```python
from build123d import *

# Parameters (mm, degrees)
F0_R     = 1.5
F1_DEPTH = 5
F2_DEPTH = 268
F3_R     = 1.65
F3_R_2   = 1.35
F4_DEPTH = 5.001
F5_W     = 12
F5_H     = 2
F6_DEPTH = 12
F7_DEPTH = 5
F8_R     = 1.65
F9_DEPTH = 52.0010001044


# Not quite as in the source:
# - an extrude ends at something that could not be found from the text; its depth is read off the source's solid


with BuildPart() as f1:
    # F0 (on Top) → F1 (new body)
    with BuildSketch(Plane.XY):
        Polygon((-52.0408339798, -45.9276453106), (-151.9144345724, -45.9276453106), (-151.9144345724, -55.9276454151), (-45.8887560524, -55.9276454151), (-25.683571109, -15.9276453106), (9.5701563833, -15.9276453106), (11.0855654276, -12.9276453106), (44.264588505, -12.9276453106), (44.264588505, -5.9276453106), (27.9570557177, -5.9276453106), (-31.8356490892, -5.9276453106), (-31.9144345724, -6.0836161342), align=None)
        with Locations((-136.9144345724, -50.9276454151)):
            Circle(F0_R, mode=Mode.SUBTRACT)
        with Locations((-96.9144345724, -50.9276454151)):
            Circle(F0_R, mode=Mode.SUBTRACT)
        with Locations((-76.9144345724, -50.9276454151)):
            Circle(F0_R, mode=Mode.SUBTRACT)
    extrude(amount=F1_DEPTH)

    # F0 (on Top) → F2 (cut, through all)
    with BuildSketch(Plane.XY):
        with Locations((-76.9144345724, -50.9276454151)):
            Circle(F0_R)
        with Locations((-96.9144345724, -50.9276454151)):
            Circle(F0_R)
    extrude(amount=-F2_DEPTH, mode=Mode.SUBTRACT)

    # F3 (on face) → F4 (cut, through all)
    with BuildSketch(Plane.XY.offset(5)):
        with Locations((39.264588505, -9.4276453106)):
            Circle(F3_R)
        with Locations((19.264588505, -9.4276453106)):
            Circle(F3_R_2)
        with Locations((-33.3638369572, -20.042586615)):
            Circle(F3_R)
        with Locations((-46.4391469312, -45.9276454151)):
            Circle(F3_R)
    extrude(amount=-F4_DEPTH, mode=Mode.SUBTRACT)

    # F5 (on face) → F6 (join)
    with BuildSketch(Plane.XY.offset(5)):
        with Locations((-58.9144345724, -54.9276454151)):
            Rectangle(F5_W, F5_H)
        with Locations((-58.9144345724, -56.9276454151)):
            Rectangle(F5_W, F5_H)
    extrude(amount=F6_DEPTH)

    # F7 (add): a face of the model
    f7_faces = [f1.faces().sort_by_distance(p)[0] for p in [
        (-58.9144345724, -56.9276454151, 5),
    ]]
    extrude(f7_faces, amount=F7_DEPTH)

    # F8 (on face) → F9 (cut, through all)
    with BuildSketch(Plane.XZ.offset(57.9276454151)):
        with Locations((-58.9144345724, 11)):
            Circle(F8_R)
    extrude(amount=-F9_DEPTH, mode=Mode.SUBTRACT)


solid = f1.part
```
Model file for the job. Use its own axes, mm. A direction names the side the tool comes from. Give positions to 0.01 mm unless a question says otherwise; leave off trailing zeros. Order: outer loops, then holes, each group sorted by start corner. A loop starts at its lowest first (then second) coordinate and runs counter-clockwise, first axis right, second up.
1) Pin check, flat tips, straight feed: pin 1 (1.5 mm diameter, centred on x = 27.5, z = 2, fed in from -Y); pin 2 (4 mm diameter, centred on y = -43.5, z = 7.5, fed in from -X); pin 3 (1.5 mm diameter, centred on x = -14.5, z = 3.5, fed in from -Y); pin 4 (2 mm diameter, centred on y = -57, z = 11.5, fed in from +X). Stop position of each tip, or through.
2) Mould opens along Y. For faces 1 (the flat face through (-49, -55.928, 2)), 2 (the flat face through (7, -5.928, 2)), 3 (the cylindrical face through (-48.088, -45.855, 2.535)) say: +Y half, -Y half, draft (parallel to the pull), parting line (faces both ways), or undercut.
3) Saw through at A-A, the plane z = 11. Write the cut outline in (x, y), then the cut area to 3 significant figures.
4) Saw through at C-C, the plane x = -18.5. Write the cut outline in (y, z), then the cut area to 3 significant figures.
5) Saw through at D-D, the plane y = -27. Write the cut outline in (x, z).
6) 3-axis set-ups, long thin cutter, end or side, ignore diameter. For faces 4 (the flat face through (-59, -56, 17)), 5 (the flat face through (27, -12.928, 2)), 6 (the flat face through (-109, -55.928, 2)), 7 (the cylindrical face through (-34.67, -21.05, 2.54)), 8 (the flat face through (-101, -45.928, 2)): which of +Z, -Z, +X, -X, +Y, -Y reach the whole face in a straight line?
7) Wall check: probe 1 along Z at (x, y) = (-102, -46); probe 2 along X at (y, z) = (-54, 15.5); probe 3 along Y at (x, z) = (-55, 10.25). Give the ranges that are in metal, low to high.
8) Saw through at B-B, the plane z = 2.75. Write the cut outline in (x, y).
Computed:
1. pin 1: stops at y = -12.93
1. pin 2: passes through
1. pin 3: stops at y = -15.93
1. pin 4: stops at x = -52.91
2. face 1: -Y half
2. face 2: +Y half
2. face 3: undercut
3. outline: (-64.91, -57.93) - (-60.56, -57.93) - (-60.56, -53.93) - (-64.91, -53.93) - close; (-57.26, -57.93) - (-52.91, -57.93) - (-52.91, -53.93) - (-57.26, -53.93) - close
3. area: 34.8 mm2
4. outline: (-15.93, 0) - (-5.93, 0) - (-5.93, 5) - (-15.93, 5) - close
4. area: 50.0 mm2
5. outline: (-42.48, 0) - (-31.28, 0) - (-31.28, 5) - (-42.48, 5) - close
6. face 4: +Z, +X, -X, +Y, -Y
6. face 5: +Z, -Z, +X, -Y
6. face 6: +Z, -Z, -X, -Y
6. face 7: +Z, -Z
6. face 8: +Z, -Z, -X, +Y
7. probe 1: z = 0 to 5
7. probe 2: x = -64.91 to -52.91
7. probe 3: y = -57.93 to -53.93
8. outline: (-151.91, -55.93) - (-64.91, -55.93) - (-64.91, -57.93) - (-52.91, -57.93) - (-52.91, -55.93) - (-45.89, -55.93) - (-25.68, -15.93) - (9.57, -15.93) - (11.09, -12.93) - (44.26, -12.93) - (44.26, -5.93) - (-31.84, -5.93) - (-52.04, -45.93) - (-151.91, -45.93) - close; hole circle Ø3 at (-136.91, -50.93); hole circle Ø3 at (-96.91, -50.93); hole circle Ø3 at (-76.91, -50.93); hole circle Ø3.3 at (-46.44, -45.93); hole circle Ø3.3 at (-33.36, -20.04); hole circle Ø2.7 at (19.26, -9.43); hole circle Ø3.3 at (39.26, -9.43)
